from build123d import *

# Parameters (mm, degrees)
F1_DEPTH = 600
F2_R     = 4
F3_DEPTH = 3.001
F5_DEPTH = 3.001


with BuildPart() as f1:
    # F0 (on Top) → F1 (new body)
    with BuildSketch(Plane.XY):
        Polygon((33, 0), (0, 0), (0, -50), (3, -50), (3, -3), (33, -3), align=None)
    extrude(amount=F1_DEPTH)

    # F2 (on face) → F3 (cut, through all)
    with BuildSketch(Plane.XZ.offset(3)):
        with Locations((18, 150)):
            Circle(F2_R)
        with Locations((18, 300)):
            Circle(F2_R)
        with Locations((18, 450)):
            Circle(F2_R)
    extrude(amount=-F3_DEPTH, mode=Mode.SUBTRACT)

    # F4 (on face) → F5 (cut, through all)
    with BuildSketch(Plane.YZ.offset(3)):
        with BuildLine():
            Line((-21.5, 506), (-31.5, 506))
            ThreePointArc((-31.5, 506), (-37.5, 500), (-31.5, 494))
            Line((-31.5, 494), (-21.5, 494))
            ThreePointArc((-21.5, 494), (-15.5, 500), (-21.5, 506))
        make_face()
        with BuildLine():
            Line((-21.5, 356), (-31.5, 356))
            ThreePointArc((-31.5, 356), (-37.5, 350), (-31.5, 344))
            Line((-31.5, 344), (-21.5, 344))
            ThreePointArc((-21.5, 344), (-15.5, 350), (-21.5, 356))
        make_face()
        with BuildLine():
            Line((-21.5, 206), (-31.5, 206))
            ThreePointArc((-31.5, 206), (-37.5, 200), (-31.5, 194))
            Line((-31.5, 194), (-21.5, 194))
            ThreePointArc((-21.5, 194), (-15.5, 200), (-21.5, 206))
        make_face()
    extrude(amount=-F5_DEPTH, mode=Mode.SUBTRACT)


solid = f1.part
Input: part model. Units: mm. Frame: model coordinates. A direction names the side the tool comes from. Give positions to 0.01 mm unless a question says otherwise; leave off trailing zeros. Loops run counter-clockwise (first coordinate to the right, second up) from the corner with the lowest first, then second, coordinate; pieces in that order, holes last. Notation, with made-up numbers: M 19.25,-15 L 68.25,-15 A15 cw 68.25,13 Z; hole C 67.25,19 d5. An arc over 180 degrees is marked long. Use CSV: the item, a comma, the result in double quotes.
(1) Section A-A, the plane z = 200. Return loops of the section in (x, y), plus the area to 3 significant figures.
Outcome:
outline,"M 0,-50 L 3,-50 L 3,-37.5 L 0,-37.5 Z; M 0,-15.5 L 3,-15.5 L 3,-3 L 33,-3 L 33,0 L 0,0 Z"
area,"174 mm²"
(2) Material intervals for L1, parallel to Z at x = 18, y = -0.6; L2, parallel to X at y = -1.8, z = 300; L3, parallel to X at y = -34.5, z = 534, sorted ascending. Write a range as [from, to].
Outcome:
L1,"z = [0, 146], [154, 296], [304, 446], [454, 600]"
L2,"x = [0, 14], [22, 33]"
L3,"x = [0, 3]"
(3) Set-up query: faces 1 (the face through (17.8, -3, 295.8)), 2 (the face through (2, -17, 600)). Return all of +Z, -Z, +X, -X, +Y, -Y with unobstructed straight access to the full face (end or side cutting, diameter ignored); none if empty.
Outcome:
face 1,"+Z, -Z, +X, -Y"
face 2,"+Z, +X, -X, +Y, -Y"
(4) Pin query (flat end, axial travel): P1, Ø1, axis at y = -41, z = 256, coming from the +X side. Return the tip coordinate at first contact, or that it passes through.
Outcome:
P1,"stops at x = 3"
